Print and shaded views of the part. All mm, measured from the part's lowest x, y and z. A direction names the side the tool comes from. Coordinates: 2 decimals unless noted, no trailing zeros. Order: outer loops, then holes, each group sorted by start corner. A loop starts at its lowest first (then second) coordinate and runs counter-clockwise, first axis right, second up. Notation, with made-up numbers: M 35,27.25 L 50,27.25 A27 cw 50,50.25 Z; hole C -15.75,-20.5 d9. An arc over 180 degrees is marked long. One line per item, written item: value.
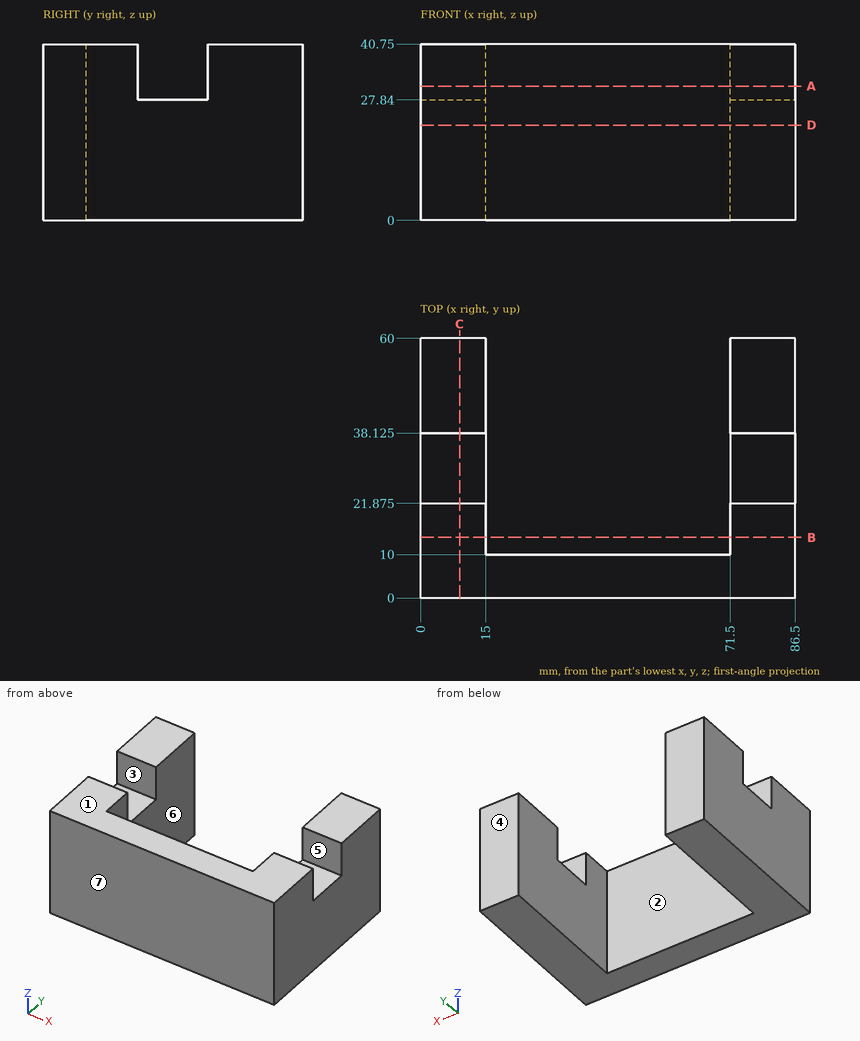
Q1. Drill centre lines: line 1 along Y through (x, z) = (82, 37) (3 decimals); line 2 along X through (y, z) = (21.5, 24); line 3 along Z through (x, y) = (6, 26.5). Where is each one in solid material? Low to high.
Recorded:
line 1: y = 0 to 21.875, 38.125 to 60
line 2: x = 0 to 15, 71.5 to 86.5
line 3: z = 0 to 27.84
Q2. Slice it at C-C (x = 9). List the corners of the cut face in (y, z) (3 decimals).
Recorded:
outline: M 0,0 L 60,0 L 60,40.75 L 38.125,40.75 L 38.125,27.84 L 21.875,27.84 L 21.875,40.75 L 0,40.75 Z
Q3. Slice it at A-A (z = 31). List the corners of the cut face in (x, y) (3 decimals).
Recorded:
outline: M 0,0 L 86.5,0 L 86.5,21.875 L 71.5,21.875 L 71.5,10 L 15,10 L 15,21.875 L 0,21.875 Z; M 0,38.125 L 15,38.125 L 15,60 L 0,60 Z; M 71.5,38.125 L 86.5,38.125 L 86.5,60 L 71.5,60 Z
Q4. Pin check, flat tips, straight feed: pin 1 Ø10 at (x, z) = (38, 17.5) entering from +Y; pin 2 Ø8 at (y, z) = (29, 31) entering from -X; pin 3 Ø12 at (x, y) = (82.5, 29) entering from +Z. Stop position of each tip, or through.
Recorded:
pin 1: stops at y = 10
pin 2: stops at x = 0
pin 3: stops at z = 27.84
Q5. Slice it at B-B (y = 14). List the corners of the cut face in (x, z).
Recorded:
outline: M 0,0 L 15,0 L 15,40.75 L 0,40.75 Z; M 71.5,0 L 86.5,0 L 86.5,40.75 L 71.5,40.75 Z
Q6. Which spindle directions (+Z, -Z, +X, -X, +Y, -Y) get a long thin tool onto all of the face, cutting with end or side? Do the marked faces 1, 2 and 3. Say none if no direction does.
Recorded:
face 1: +Z, +X, -X, +Y, -Y
face 2: +Z, -Z, +Y
face 3: +Z, +X, -X
Q7. Mould opens along Y. For the marked faces 4, 5, 6 and 7 say: released by +Y, released by -Y, zero draft, split by the parting line, or undercut.
Recorded:
face 4: released by +Y
face 5: undercut
face 6: zero draft
face 7: released by -Y
Q8. Slice it at D-D (z = 22). List the corners of the cut face in (x, y).
Recorded:
outline: M 0,0 L 86.5,0 L 86.5,60 L 71.5,60 L 71.5,10 L 15,10 L 15,60 L 0,60 Z
